from build123d import *

# Parameters (mm, degrees)
F0_R     = 75.1711608748
F0_R_2   = 20.15
F1_DEPTH = 13


# Not quite as in the source:
# - a feature names something its author has since deleted; it is built from what else it names
# - the program builds the solid bodies; features that only make, move or delete a surface that nothing else refers to are left out


with BuildPart() as f1:
    # F0 (on Front) → F1 (new body)
    with BuildSketch(Plane.XZ):
        Circle(F0_R)
        with Locations((0, -44.8568575084)):
            Circle(F0_R_2, mode=Mode.SUBTRACT)
        with Locations((-45.5452017486, 0)):
            Circle(F0_R_2, mode=Mode.SUBTRACT)
        with Locations((45.3157536685, 0)):
            Circle(F0_R_2, mode=Mode.SUBTRACT)
        with Locations((0, 44.6274131536)):
            Circle(F0_R_2, mode=Mode.SUBTRACT)
    extrude(amount=F1_DEPTH)

    # F2 (on Top) → F3 (revolve)
    with BuildSketch(Plane.XY):
        with BuildLine():
            Line((-21.1639329791, 0), (0, 0))
            Line((0, 0), (0, 80.0915658474))
            Line((0, 80.0915658474), (-21.1639329791, 80.0915658474))
            add(Edge.make_bspline(
                [(-21.1639329791, 0), (-19.2742553322, 4.6189694115), (3.1468380819, 14.4620732239), (-34.8000145769, 30.7354101763), (8.134922476, 47.7855342492), (-36.319607523, 61.0135638885), (9.834598536, 75.0191615104), (-16.6499702233, 77.9874063736), (-21.1639329791, 80.0915658474)],
                knots=[0, 0, 0, 0, 0.1626396624, 0.3304383742, 0.5058929878, 0.6723966985, 0.8424869218, 1, 1, 1, 1], degree=3))
        make_face()
    revolve(axis=Axis((0, 40.0457829237, 0), (0, 1, 0)))


solid = f1.part
Input: part model. Units: mm. Frame: model coordinates. A direction names the side the tool comes from. Round coordinates to 2 decimals unless told otherwise and drop trailing zeros. Order: outer loops, then holes, each group sorted by start corner. A loop starts at its lowest first (then second) coordinate and runs counter-clockwise, first axis right, second up.
1. Set-up query: faces 4 (the face through (16, 0, -16)), 5 (the face through (0, 80.092, 0)). Return all of +Z, -Z, +X, -X, +Y, -Y with unobstructed straight access to the full face (end or side cutting, diameter ignored); none if empty.
The answers:
face 4: +Y
face 5: +Z, -Z, +X, -X, +Y
2. Cut plane B-B, the plane x = 46.5. Output: boundary loops of the cut face in (y, z).
The answers:
outline: (-13, -59.06) - (0, -59.06) - (0, -20.12) - (-13, -20.12) - close; (-13, 20.12) - (0, 20.12) - (0, 59.06) - (-13, 59.06) - close
3. Material intervals for line 1 (Z direction, x = 0, y = -3.25); line 2 (Y direction, x = -12, z = 10.5); line 3 (Y direction, x = 62, z = -37), sorted ascending.
The answers:
line 1: z = -75.17 to -65.01, -24.71 to 24.48, 64.78 to 75.17
line 2: y = -13 to 5.55, 23.04 to 37.24, 55.51 to 66.22, 78.45 to 80.09
line 3: y = -13 to 0
4. Mould query, pull axis X, two halves, no side actions, for faces 1 (the face through (-59.653, -6.409, -45.74)), 2 (the face through (9.3, -6.41, 26.75)), 3 (the face through (-1, -13, 1)). Classes: released by +X, released by -X, zero draft, split by the parting line, or undercut.
The answers:
face 1: split by the parting line
face 2: undercut
face 3: zero draft
5. Cut plane C-C, the plane x = 0. State how many separate pieces and enclosed holes the cut face has, then the cut area to 3 significant figures.
The answers:
separate pieces: 3
enclosed holes: 0
area: 3,130 mm2
6. Cut plane A-A, the plane z = 47.5. Output: boundary loops of the cut face in (x, y).
The answers:
outline: (-58.26, -13) - (-19.94, -13) - (-19.94, 0) - (-58.26, 0) - close; (19.94, -13) - (58.26, -13) - (58.26, 0) - (19.94, 0) - close
